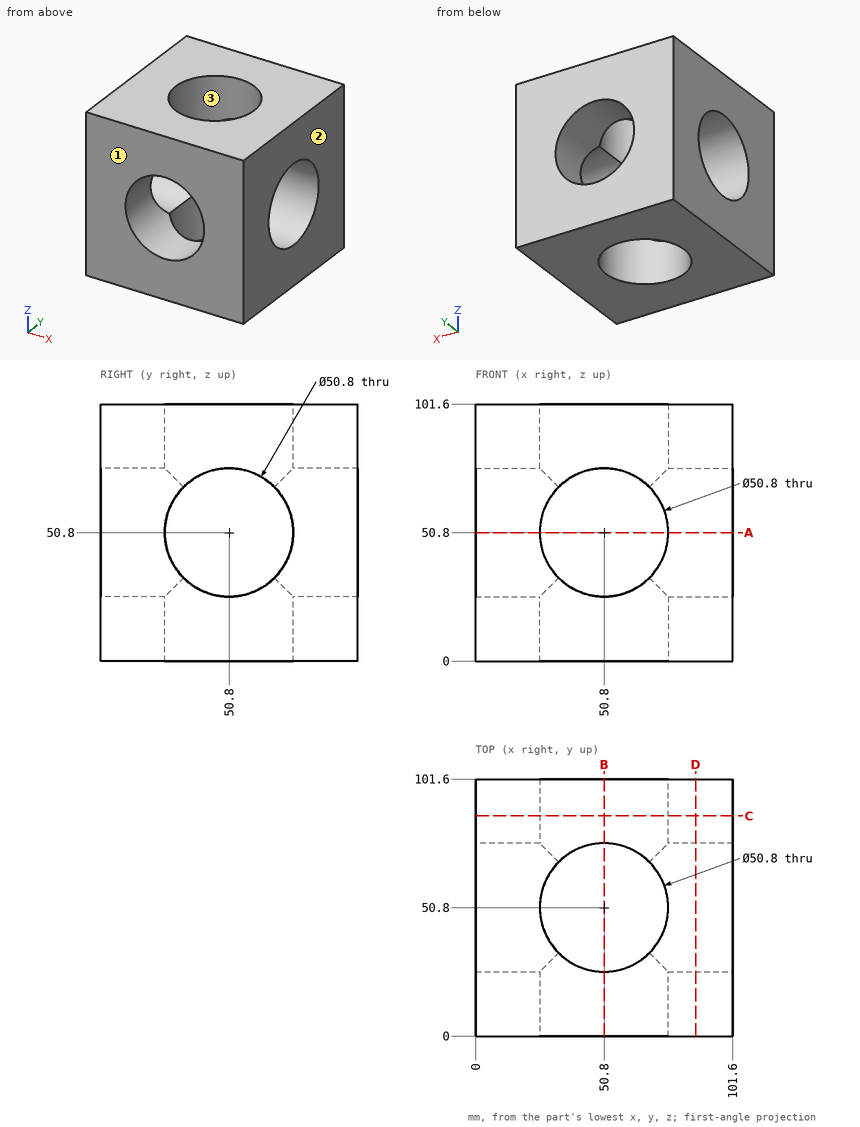
Design review of the part shown in the three views and the two pictorial views. Dimensions are in mm from the part's minimum x, y and z. Give positions to 0.01 mm unless a question says otherwise; leave off trailing zeros. Loops run counter-clockwise (first coordinate to the right, second up) from the corner with the lowest first, then second, coordinate; pieces in that order, holes last. Notation, with made-up numbers: (13.25, 23) -> (67.25, 23) arc R4 cw to (67.25, 30) -> close; hole circle Ø1 at (0.25, -2.5). An arc over 180 degrees is marked (long way). Put each result on its own line as item: value. Start each with the question number.
1. Clearance check with flat-ended pins moving along their axes: P1, Ø4, axis at y = 30, z = 44.5, coming from the -X side; P2, Ø6, axis at x = 91, y = 91, coming from the -Z side. State where each tip first meets the part, or that it passes through.
2. Wall thickness on probe 1 along X at (y, z) = (86, 50); probe 2 along Z at (x, y) = (88, 50.8): over which ranges is each line inside the solid? List them lowest first.
3. Mouldability with a two-part tool opening along X and no side actions: class the marked faces 1, 2 and 3 as released by +X, released by -X, zero draft, split by the parting line, or undercut.
4. We need section C-C on y = 87. State the section outline as (x, z) points.
5. We need section A-A on z = 50.8. State the section outline as (x, y) points, then the cut area to 3 significant figures.
Determined:
1. P1: through
1. P2: z = 0
2. probe 1: 0 to 25.41, 76.19 to 101.6
2. probe 2: 0 to 25.4, 76.2 to 101.6
3. face 1: zero draft
3. face 2: released by +X
3. face 3: undercut
4. outline: (0, 0) -> (101.6, 0) -> (101.6, 101.6) -> (0, 101.6) -> close; hole circle Ø50.8 at (50.8, 50.8)
5. outline: (0, 0) -> (25.4, 0) -> (25.4, 25.4) -> (0, 25.4) -> close; (0, 76.2) -> (25.4, 76.2) -> (25.4, 101.6) -> (0, 101.6) -> close; (76.2, 0) -> (101.6, 0) -> (101.6, 25.4) -> (76.2, 25.4) -> close; (76.2, 76.2) -> (101.6, 76.2) -> (101.6, 101.6) -> (76.2, 101.6) -> close
5. area: 2,580 mm^2
